Work out the finished part from the listing and answer in its coordinate system (mm). Face numbers are marked on the shaded views. A direction names the side the tool comes from. Give positions to 0.01 mm unless a question says otherwise; leave off trailing zeros. Loops run counter-clockwise (first coordinate to the right, second up) from the corner with the lowest first, then second, coordinate; pieces in that order, holes last. Notation, with made-up numbers: M 82.5,-25.5 L 124.5,-25.5 A5 ccw 124.5,-21.5 Z; hole C 49.25,-10 d3. An arc over 180 degrees is marked long. Use a Markdown table: item, result.
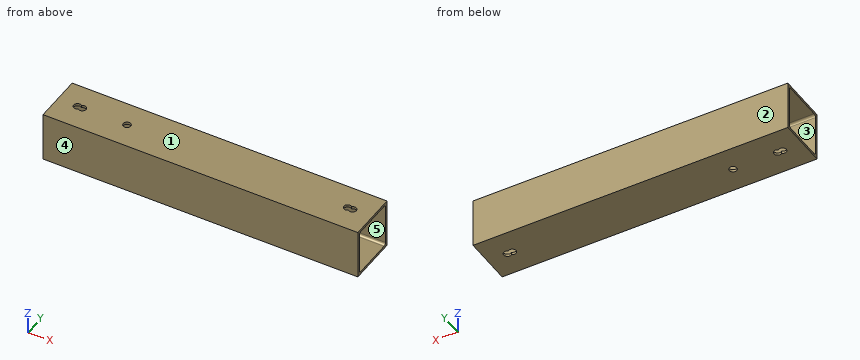
```python
from build123d import *

# Parameters (mm, degrees)
SKETCH1_W           = 20
SKETCH1_H           = 20
BOSS_EXTRUDE1_DEPTH = 127
SKETCH5_R           = 1.5
CUT_EXTRUDE4_DEPTH  = 20
SKETCH2_R           = 1.5
CUT_EXTRUDE1_DEPTH  = 600
SKETCH3_R           = 1.5
CUT_EXTRUDE2_DEPTH  = 30


with BuildPart() as part:
    # Sketch1 → Boss-Extrude1 (new body)
    with BuildSketch(Plane(origin=(0, 0, 0), x_dir=(0, 0, -1), z_dir=(1, 0, 0))):
        Rectangle(SKETCH1_W, SKETCH1_H)
        with BuildLine():
            Line((-8, -9), (8, -9))
            ThreePointArc((8, -9), (8.707106781, -8.707106781), (9, -8))
            Line((9, -8), (9, 8))
            ThreePointArc((9, 8), (8.707106781, 8.707106781), (8, 9))
            Line((8, 9), (-8, 9))
            ThreePointArc((-8, 9), (-8.707106781, 8.707106781), (-9, 8))
            Line((-9, 8), (-9, -8))
            ThreePointArc((-9, -8), (-8.707106781, -8.707106781), (-8, -9))
        make_face(mode=Mode.SUBTRACT)
    extrude(amount=BOSS_EXTRUDE1_DEPTH)

    # Sketch5 → Cut-Extrude4 (cut)
    with BuildSketch(Plane.XY.offset(10)):
        with Locations((10, 0)):
            Circle(SKETCH5_R)
        with Locations((117, 0)):
            Circle(SKETCH5_R)
    extrude(amount=-CUT_EXTRUDE4_DEPTH, mode=Mode.SUBTRACT)

    # Sketch2 → Cut-Extrude1 (cut)
    with BuildSketch(Plane.XY.offset(10)):
        with Locations((8, 0)):
            Circle(SKETCH2_R)
        with Locations((28, 0)):
            Circle(SKETCH2_R)
    extrude(amount=-CUT_EXTRUDE1_DEPTH, mode=Mode.SUBTRACT)

    # Sketch3 → Cut-Extrude2 (cut)
    with BuildSketch(Plane.XY.offset(10)):
        with Locations((119, 0)):
            Circle(SKETCH3_R)
        with Locations((139, 0)):
            Circle(SKETCH3_R)
    extrude(amount=-CUT_EXTRUDE2_DEPTH, mode=Mode.SUBTRACT)


solid = part.part
```
(1) The mould has two halves that part along Y. Classify the marked faces 1, 2 and 3: released by +Y, released by -Y, zero draft, split by the parting line, or undercut.
Entries:
| item | result |
|---|---|
| face 1 | zero draft |
| face 2 | released by +Y |
| face 3 | undercut |
(2) Consider probe 1 along Y at (x, z) = (53, 6.75); probe 2 along Y at (x, z) = (8, -9.65). Determine where each line is inside the solid, lowest interval first. Write a range as [from, to].
Entries:
| item | result |
|---|---|
| probe 1 | y = [-10, -9], [9, 10] |
| probe 2 | y = [-10, -1.5], [1.5, 10] |
(3) Which of the six approach directions +Z, -Z, +X, -X, +Y, -Y give full straight-line access (tool end or side, diameter ignored) to the marked faces 4 and 5?
Entries:
| item | result |
|---|---|
| face 4 | +Z, -Z, +X, -X, -Y |
| face 5 | +X, -X |
(4) A cutting plane is placed at A-A (z = 2). Write down the section's boundary in (x, y), and give its area (3 significant figures).
Entries:
| item | result |
|---|---|
| outline | M 0,-10 L 127,-10 L 127,-9 L 0,-9 Z; M 0,9 L 127,9 L 127,10 L 0,10 Z |
| area | 254 mm² |
(5) A cutting plane is placed at D-D (x = 89.5). Write down the section's boundary in (y, z).
Entries:
| item | result |
|---|---|
| outline | M -10,-10 L 10,-10 L 10,10 L -10,10 Z; hole M -9,-8 A1 ccw -8,-9 L 8,-9 A1 ccw 9,-8 L 9,8 A1 ccw 8,9 L -8,9 A1 ccw -9,8 Z |
(6) A cutting plane is placed at C-C (x = 28). Write down the section's boundary in (y, z).
Entries:
| item | result |
|---|---|
| outline | M -10,-10 L -1.5,-10 L -1.5,-9 L -8,-9 A1 cw -9,-8 L -9,8 A1 cw -8,9 L -1.5,9 L -1.5,10 L -10,10 Z; M 1.5,-10 L 10,-10 L 10,10 L 1.5,10 L 1.5,9 L 8,9 A1 cw 9,8 L 9,-8 A1 cw 8,-9 L 1.5,-9 Z |
